Autodesk Inventor part; units mm, degrees
ref_plane "YZ Plane" through (0, 0, 0) normal (1, 0, 0) x (0, 1, 0)
ref_plane "XZ Plane" through (0, 0, 0) normal (0, 1, 0) x (-1, 0, 0)
ref_plane "XY Plane" through (0, 0, 0) normal (0, 0, 1) x (1, 0, 0)
sketch "Sketch1" plane through (0, 0, 0) normal (0, 0, 1) x (1, 0, 0)
  line L0 (-61.6808, 42.3688) -> (58.3192, 42.3688)
  line L1 (58.3192, 42.3688) -> (58.3192, -7.6312)
  line L2 (58.3192, -7.6312) -> (-61.6808, -7.6312)
  line L3 (-61.6808, -7.6312) -> (-61.6808, 42.3688)
  dimension "d0" = 50
  dimension "d1" = 120
extrude "Plate1" add sketch "Sketch1" along normal blind 0.5
sketch "Sketch2" plane through (0, 0, 0.5) normal (0, 0, 1) x (1, 0, 0)
  line L0 (-12.7986, 24.2423) -> (7.2014, 24.2423)
  line L1 (7.2014, 24.2423) -> (7.2014, 16.2423)
  line L2 (7.2014, 16.2423) -> (-12.7986, 16.2423)
  line L3 (-12.7986, 16.2423) -> (-12.7986, 24.2423)
  point P0 (-2.7986, 20.2423)
  dimension "LG_G" = 20
  dimension "LT_G" = 8
  dimension "d21" = 4
  dimension "d22" = 10
extrude "Extrusion1" add sketch "Sketch2" against normal blind 1.5
sketch "Sketch3" plane through (0, 0, 0.5) normal (0, 0, 1) x (1, 0, 0)
  line L0 (-12.7986, 24.2423) -> (7.2014, 24.2423)
  line L1 (-12.7986, 16.2423) -> (-12.7986, 24.2423)
  line L2 (7.2014, 16.2423) -> (-12.7986, 16.2423)
  line L3 (7.2014, 24.2423) -> (7.2014, 16.2423)
  line L4 (-12.2986, 24.2423) -> (6.7014, 24.2423)
  line L5 (6.7014, 24.2423) -> (6.7014, 16.2423)
  line L6 (6.7014, 16.2423) -> (-12.2986, 16.2423)
  line L7 (-12.2986, 16.2423) -> (-12.2986, 24.2423)
  dimension "d9" = 0.5
  dimension "d10" = 0.5
extrude "Extrusion2" cut sketch "Sketch3" against normal blind 1 contours L0 L5 L2 L7
sketch "Sketch4" plane through (0, 0, 0.5) normal (0, 0, 1) x (1, 0, 0)
  line L0 (-12.7986, 24.2423) -> (7.2014, 24.2423)
  line L1 (-12.7986, 16.2423) -> (-12.7986, 24.2423)
  line L2 (7.2014, 24.2423) -> (7.2014, 16.2423)
  line L3 (7.2014, 16.2423) -> (-12.7986, 16.2423)
  line L4 (-13.2986, 24.7423) -> (7.7014, 24.7423)
  line L5 (7.7014, 24.7423) -> (7.7014, 24.2423)
  line L6 (7.7014, 24.2423) -> (-13.2986, 24.2423)
  line L7 (-13.2986, 24.2423) -> (-13.2986, 24.7423)
  line L8 (-13.2986, 16.2423) -> (7.7014, 16.2423)
  line L9 (7.7014, 16.2423) -> (7.7014, 15.7423)
  line L10 (7.7014, 15.7423) -> (-13.2986, 15.7423)
  line L11 (-13.2986, 15.7423) -> (-13.2986, 16.2423)
  line L12 (6.7014, 16.2423) -> (-12.2986, 16.2423)
  dimension "d13" = 0.5
  dimension "d14" = 0.5
  dimension "d15" = 0.5
  dimension "d16" = 0.5
extrude "Cut1" cut sketch "Sketch4" against normal blind 0.5 contours L6 L7 L4 L5 L0 | L3 L8 L9 L10 L11
fillet "Fillet1" radius 0.8 4 edges at (-12.2986, 20.2423, 0.5) (6.7014, 20.2423, 0.5) (-12.7986, 20.2423, -1) (7.2014, 20.2423, -1)
fillet "Fillet2" radius 0.3 4 edges at (7.2014, 20.2423, 0) (-12.7986, 20.2423, 0) (-12.2986, 20.2423, -0.5) (6.7014, 20.2423, -0.5)
equation "\"d7\" = 3 * Thickness"
equation "\"d9\" = Thickness"
equation "\"d10\" = Thickness"
equation "\"d11\" = 2 * Thickness"
equation "\"d13\" = Thickness"
equation "\"d14\" = Thickness"
equation "\"d15\" = Thickness"
equation "\"d16\" = Thickness"
equation "\"d17\" = Thickness"
equation "\"d2\" = Thickness"
equation "\"BendRadius\" = Thickness"
equation "\"BendReliefWidth\" = Thickness"
equation "\"BendReliefDepth\" = 0.5 * Thickness"
equation "\"CornerReliefSize\" = 4 * Thickness"
equation "\"MinimumRemnant\" = 2 * Thickness"
equation "\"TransitionRadius\" = BendRadius"
equation "\"JacobiRadiusSize\" = BendRadius"
equation "\"GapSize\" = Thickness"
properties part number "DecupajAgatare1"
For this review, take the finished solid that the model builds, in its own axes (mm). A direction names the side the tool comes from. Coordinates: 2 decimals unless noted, no trailing zeros. Write each loop counter-clockwise with the first axis right and the second up, starting at its lowest first coordinate (ties: lowest second). Pieces come first, ordered by that corner, then holes. Notation, with made-up numbers: (42.5, 82.25) -> (77.5, 82.25) arc R22 ccw to (77.5, 111.25) -> close; hole circle Ø4 at (-33.5, 81.5). An arc over 180 degrees is marked (long way). Write each question's results on one line, items separated by ' | '. Start each with the question number.
1) Insertion check: pin 1 (2.5 mm diameter, centred on x = 1, y = 22, fed in from +Z); pin 2 (15 mm diameter, centred on x = 17, y = 19, fed in from -Z). Each pin has a flat end and moves straight along its axis. Give the tip position at first contact, or say it passes through.
2) Consider section C-C (x = 27.5). Write out the cut boundary in (y, z).
3) Consider section A-A (x = -6.5). Write out the cut boundary in (y, z), plus the area to 3 significant figures.
4) For faces 1 (the face through (-3, 20, -0.5)), 2 (the face through (-3, 20, -1)), list the 3-axis set-ups (+Z, -Z, +X, -X, +Y, -Y) from which the entire face can be reached by the end or side of a thin tool; tool diameter is ignored.
5) Wall thickness on L1, parallel to Y at x = -12, z = 0.05; L2, parallel to Z at x = 41, y = 0.5; L3, parallel to X at y = 23.5, z = 0.05: over which ranges is each line inside the solid? List them lowest first. Write a range as [from, to].
6) Consider section B-B (y = 36.5). Write out the cut boundary in (x, z).
Geometry says:
1) pin 1: z = -0.5 | pin 2: z = 0
2) outline: (-7.63, 0) -> (42.37, 0) -> (42.37, 0.5) -> (-7.63, 0.5) -> close
3) outline: (-7.63, 0) -> (15.74, 0) -> (15.74, 0.5) -> (-7.63, 0.5) -> close; (16.24, -1) -> (24.24, -1) -> (24.24, -0.5) -> (16.24, -0.5) -> close; (24.74, 0) -> (42.37, 0) -> (42.37, 0.5) -> (24.74, 0.5) -> close | area: 24.5 mm^2
4) face 1: +Z, +Y, -Y | face 2: -Z, +X, -X, +Y, -Y
5) L1: [-7.63, 15.74], [24.74, 42.37] | L2: [0, 0.5] | L3: [-61.68, -12.38], [6.78, 58.32]
6) outline: (-61.68, 0) -> (58.32, 0) -> (58.32, 0.5) -> (-61.68, 0.5) -> close
